Design review of the part built by this model. Coordinates are the model's own, in mm. Coordinates: 2 decimals unless noted, no trailing zeros. Loops run counter-clockwise (first coordinate to the right, second up) from the corner with the lowest first, then second, coordinate; pieces in that order, holes last. Notation, with made-up numbers: (54.5, 15) -> (99.5, 15) arc R21 ccw to (99.5, 36) -> close; hole circle Ø6 at (59.25, -17). An arc over 180 degrees is marked (long way). Use a Markdown table: item, result. Add a question column.
Q1. Take a section at A-A on x = 0. Write out the cut boundary in (y, z), plus the area to 3 significant figures.
Q2. For probe 1 along Z at (x, y) = (0, 0.8); probe 2 along Z at (x, y) = (-0.75, 1.3); probe 3 along X at (y, z) = (1.2, -56.5), list the stretches that pass through material, from the lowest coordinate up.
Q3. Take a section at B-B on y = 0.55. Write out the cut boundary in (x, z).
Q4. Take a section at D-D on x = 15. Write out the cut boundary in (y, z).
Q5. Take a section at C-C on z = -43. Write out the cut boundary in (x, y), plus the area to 3 significant figures.
Autodesk Inventor part; units mm, degrees
ref_plane "YZ Plane" through (0, 0, 0) normal (1, 0, 0) x (0, 1, 0)
ref_plane "XZ Plane" through (0, 0, 0) normal (0, 1, 0) x (-1, 0, 0)
ref_plane "XY Plane" through (0, 0, 0) normal (0, 0, 1) x (1, 0, 0)
sketch "Sketch1" plane through (0, 0, 0) normal (0, 1, 0) x (-1, 0, 0)
  circle A0 centre (0, 0) radius 4
  line L0 (2, -5) -> (2, -51.029)
  line L1 (-2, -7.543) -> (-2, -44.0823)
  circle A1 centre (0, -56.029) radius 4
  circle A2 centre (-20.6662, -18.892) radius 4
  line L2 (-4.2179, -6.5655) -> (-15.9345, -17.2762)
  line L3 (-4.9298, -1.7969) -> (-18.4353, -14.1429)
  line L4 (-16.6903, -21.9238) -> (-4.0616, -44.6173)
  line L5 (-20.1855, -23.8688) -> (-3.976, -52.9972)
  arc A3 (2.8966, -2.7586) -> (2, -5) centre (5.25, -5) ccw
  arc A4 (2, -51.029) -> (2.8966, -53.2704) centre (5.25, -51.029) ccw
  arc A5 (-4.9298, -1.7969) -> (-3.9954, 0.1924) centre (-6.875, 0.331) ccw
  arc A6 (-20.5001, -14.8954) -> (-18.4353, -14.1429) centre (-20.3803, -12.0152) ccw
  line L6 (0, 0) -> (-20.6662, -18.892) construction
  line L7 (-20.6662, -18.892) -> (0, -56.029) construction
  arc A7 (-15.9345, -17.2762) -> (-16.6663, -18.9207) centre (-14.4164, -18.9369) ccw
  arc A8 (-16.8633, -20.1321) -> (-16.6903, -21.9238) centre (-14.7242, -20.8297) ccw
  arc A9 (-2, -7.543) -> (-4.2179, -6.5655) centre (-3.3243, -7.543) ccw
  arc A10 (-4.0616, -44.6173) -> (-2, -44.0823) centre (-3.1002, -44.0823) ccw
  arc A11 (-20.1855, -23.8688) -> (-21.6168, -22.7774) centre (-22.1516, -24.9629) ccw
  arc A12 (-3.8029, -54.7889) -> (-3.976, -52.9972) centre (-5.942, -54.0913) ccw
  point P0 (-21.4801, -12.8095)
  dimension "d0" = 8
  dimension "d1" = 8
  dimension "d2" = 8
  dimension "d4" = 42.5
  dimension "d5" = 28
  dimension "d6" = 2
  dimension "d7" = 2
  dimension "d8" = 5
  dimension "d10" = 5
  dimension "d11" = 0
  dimension "d12" = 5.2471
  dimension "d14" = 5.247
  dimension "d15" = 2
  dimension "d16" = 2
  dimension "d17" = 2
  dimension "d18" = 2
  dimension "d19" = 4
  dimension "d20" = 5
  dimension "d21" = 5
  dimension "d22" = 5
  dimension "d23" = 1.1002
  dimension "d24" = 1.3243
  dimension "d38" = 56.029
extrude "Extrusion1" add sketch "Sketch1" along normal blind 4 contours A0 | A2 | A1
extrude "Extrusion2" add sketch "Sketch1" along normal blind 1.7 contours A0 A3 L0 A4 A1 A12 L5 A11 A2 A8 L4 A10 L1 A9 L2 A7 A6 L3 A5 | A7 L2 A9 L1 A10 L4 A8 A2
sketch "Sketch2" plane through (0, 4, 0) normal (0, 1, 0) x (1, 0, 0)
  circle A0 centre (0, 0) radius 4
  circle A1 centre (0, 0) radius 1.5
  circle A2 centre (20.6662, 18.892) radius 4
  circle A3 centre (20.6662, 18.892) radius 1.5
  circle A4 centre (0, 56.029) radius 1.5
  circle A5 centre (0, 56.029) radius 4
  dimension "d29" = 3
  dimension "d30" = 3
  dimension "d31" = 3
  dimension "d36" = 0
extrude "Extrusion3" cut sketch "Sketch2" against normal blind 4 contours A1 | A3 | A4
sketch "Sketch3" plane through (-2, 0, -51.029) normal (-1, 0, 0) x (0, 0, 1)
  line L0 (60.4555, 1.7) -> (-13.4083, 1.7)
  line L1 (-13.4083, 1.7) -> (-13.4083, 27.1644)
  line L2 (-13.4083, 27.1644) -> (60.4555, 27.1644)
  line L3 (60.4555, 27.1644) -> (60.4555, 1.7)
  point P0 (51.029, 0)
extrude "Extrusion4" cut sketch "Sketch3" along normal mid plane 100
equation "\"BendRadius\" = Thickness"
equation "\"BendReliefWidth\" = Thickness"
equation "\"BendReliefDepth\" = 0.5 * Thickness"
equation "\"CornerReliefSize\" = 4 * Thickness"
equation "\"MinimumRemnant\" = 2 * Thickness"
equation "\"TransitionRadius\" = BendRadius"
equation "\"JacobiRadiusSize\" = BendRadius"
equation "\"GapSize\" = Thickness"
properties part number "A2P2"
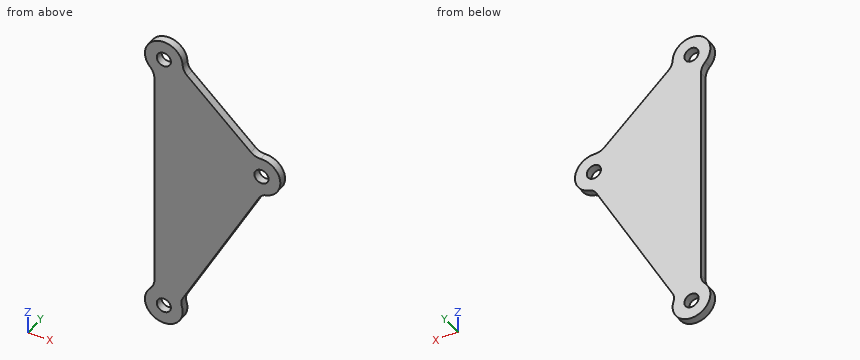
Answer list:
| question | item | result |
|---|---|---|
| 1 | outline | (0, -60.03) -> (1.7, -60.03) -> (1.7, -57.53) -> (0, -57.53) -> close; (0, -54.53) -> (1.7, -54.53) -> (1.7, -1.5) -> (0, -1.5) -> close; (0, 1.5) -> (1.7, 1.5) -> (1.7, 4) -> (0, 4) -> close |
| 1 | area | 98.6 mm² |
| 2 | probe 1 | -60.03 to -57.53, -54.53 to -1.5, 1.5 to 4 |
| 2 | probe 2 | -59.96 to -57.33, -54.73 to -1.3, 1.3 to 3.93 |
| 2 | probe 3 | -3.97 to -1.42, 1.42 to 3.97 |
| 3 | outline | (-2.9, -53.27) arc R4 ccw (long way) to (3.8, -54.79) arc R2.25 cw to (3.98, -53) -> (20.19, -23.87) arc R2.25 cw to (21.62, -22.78) arc R4 ccw to (20.5, -14.9) arc R2.88 cw to (18.44, -14.14) -> (4.93, -1.8) arc R2.88 cw to (4, 0.19) arc R4 ccw (long way) to (-2.9, -2.76) arc R3.25 cw to (-2, -5) -> (-2, -51.03) arc R3.25 cw to start; hole circle Ø3 at (0, -56.03); hole circle Ø3 at (0, 0); hole circle Ø3 at (20.67, -18.89) |
| 4 | outline | (0, -33.19) -> (1.7, -33.19) -> (1.7, -11) -> (0, -11) -> close |
| 5 | outline | (-2, 0) -> (9.54, 0) -> (9.54, 1.7) -> (-2, 1.7) -> close |
| 5 | area | 19.6 mm² |
